The model under review builds one solid part; all positions refer to its coordinate system, in mm. A direction names the side the tool comes from. Coordinates: 2 decimals unless noted, no trailing zeros. Order: outer loops, then holes, each group sorted by start corner. A loop starts at its lowest first (then second) coordinate and runs counter-clockwise, first axis right, second up. Notation, with made-up numbers: (-12, 80.25) - (42, 80.25) arc R17 cw to (42, 94.25) - close; hole circle Ø6 at (9, -6). An arc over 180 degrees is marked (long way). Answer in a Markdown table with one row per item.
```python
from build123d import *

# Parameters (mm, degrees)
ESQUISSE1_W              = 57.9
ESQUISSE1_H              = 86
BOSS_EXTRU_1_DEPTH       = 80
ESQUISSE2_W              = 49.9
ESQUISSE2_H              = 78
ENL_V_MAT_EXTRU_1_DEPTH  = 75
ESQUISSE3_W              = 10
ESQUISSE3_H              = 10
BOSS_EXTRU_2_DEPTH       = 10
ESQUISSE4_R              = 2.75
ENL_V_MAT_EXTRU_2_DEPTH  = 5.85
ESQUISSE47_R             = 2.25
ENL_V_MAT_EXTRU_25_DEPTH = 10
ESQUISSE19_W             = 50
ESQUISSE19_H             = 20
BOSS_EXTRU_9_DEPTH       = 4.75
CONG_1_R                 = 3
ESQUISSE29_W             = 10
ESQUISSE29_H             = 5
ENL_V_MAT_EXTRU_11_DEPTH = 100.346187647
ESQUISSE32_W             = 57.9
ESQUISSE32_H             = 62.5
ENL_V_MAT_EXTRU_16_DEPTH = 4
ESQUISSE46_W             = 3
ESQUISSE46_H             = 5.5
BOSS_EXTRU_10_DEPTH      = 78
ENL_V_START              = -1.5
ENL_V_MAT_EXTRU_20_DEPTH = 11.5
ENL_V_MAT_EXTRU_21_DEPTH = 1.7
CHANFREIN1_SIZE          = 6
ESQUISSE45_R             = 2.75
ENL_V_MAT_EXTRU_24_DEPTH = 100.346187647
ESQUISSE48_W             = 8
ESQUISSE48_H             = 4
BOSS_EXTRU_11_DEPTH      = 15
ESQUISSE49_R             = 2.75
ENL_V_MAT_EXTRU_26_DEPTH = 15
CONG_2_R                 = 2


with BuildPart() as part:
    # Esquisse1 → Boss.-Extru.1 (new body)
    with BuildSketch(Plane.XY):
        Rectangle(ESQUISSE1_W, ESQUISSE1_H)
    extrude(amount=BOSS_EXTRU_1_DEPTH)

    # Esquisse2 → Enlèv. mat.-Extru.1 (cut)
    with BuildSketch(Plane.XY.offset(80)):
        Rectangle(ESQUISSE2_W, ESQUISSE2_H)
    extrude(amount=-ENL_V_MAT_EXTRU_1_DEPTH, mode=Mode.SUBTRACT)

    # Esquisse3 → Boss.-Extru.2 (add)
    with BuildSketch(Plane.XY.offset(80)):
        with Locations((-23.95, 38)):
            Rectangle(ESQUISSE3_W, ESQUISSE3_H)
        with Locations((-23.95, -38)):
            Rectangle(ESQUISSE3_W, ESQUISSE3_H)
        with Locations((23.95, -38)):
            Rectangle(ESQUISSE3_W, ESQUISSE3_H)
        with Locations((23.95, 38)):
            Rectangle(ESQUISSE3_W, ESQUISSE3_H)
    extrude(amount=-BOSS_EXTRU_2_DEPTH)

    # Esquisse4 → Enlèv. mat.-Extru.2 (cut)
    with BuildSketch(Plane.XY.offset(80)):
        with Locations((23.95, -38)):
            Circle(ESQUISSE4_R)
        with Locations((-23.95, -38)):
            Circle(ESQUISSE4_R)
        with Locations((-23.95, 38)):
            Circle(ESQUISSE4_R)
        with Locations((23.95, 38)):
            Circle(ESQUISSE4_R)
    extrude(amount=-ENL_V_MAT_EXTRU_2_DEPTH, mode=Mode.SUBTRACT)

    # Esquisse47 → Enlèv. mat.-Extru.25 (cut)
    with BuildSketch(Plane.XY.offset(80)):
        with Locations((23.95, -38)):
            Circle(ESQUISSE47_R)
        with Locations((-23.95, -38)):
            Circle(ESQUISSE47_R)
        with Locations((-23.95, 38)):
            Circle(ESQUISSE47_R)
        with Locations((23.95, 38)):
            Circle(ESQUISSE47_R)
    extrude(amount=-ENL_V_MAT_EXTRU_25_DEPTH, mode=Mode.SUBTRACT)

    # Esquisse19 → Boss.-Extru.9 (add)
    with BuildSketch(Plane(origin=(0, 0, 0), x_dir=(-1, 0, 0), z_dir=(0, 0, -1))):
        with Locations((0, -7)):
            Rectangle(ESQUISSE19_W, ESQUISSE19_H)
    extrude(amount=BOSS_EXTRU_9_DEPTH)

    # Congé1
    cong_1_edges = [part.edges().sort_by_distance(p)[0] for p in [
        (0, -17, 0),
    ]]
    fillet(cong_1_edges, radius=CONG_1_R)

    # Esquisse29 → Enlèv. mat.-Extru.11 (cut, through all)
    with BuildSketch(Plane(origin=(0, 0, -4.75), x_dir=(-1, 0, 0), z_dir=(0, 0, -1))):
        with Locations((0, -5)):
            Rectangle(ESQUISSE29_W, ESQUISSE29_H)
    extrude(amount=-ENL_V_MAT_EXTRU_11_DEPTH, mode=Mode.SUBTRACT)

    # Esquisse32 → Enlèv. mat.-Extru.16 (cut)
    with BuildSketch(Plane.XZ.offset(43)):
        with Locations((0, 33.25)):
            Rectangle(ESQUISSE32_W, ESQUISSE32_H)
    extrude(amount=-ENL_V_MAT_EXTRU_16_DEPTH, mode=Mode.SUBTRACT)

    # Esquisse46 → Boss.-Extru.10 (add)
    with BuildSketch(Plane.XZ.offset(39)):
        with Locations((-23.45, 15.75)):
            Rectangle(ESQUISSE46_W, ESQUISSE46_H)
    boss_extru_10 = extrude(amount=-BOSS_EXTRU_10_DEPTH)

    # Esquisse38 → Enlèv. mat.-Extru.20 (cut)
    with BuildSketch(Plane(origin=(-24.95, 0, 0), x_dir=(0, 0, -1), z_dir=(1, 0, 0)).offset(ENL_V_START)):
        with BuildLine():
            Line((-16.95, -39), (-16.95, 36))
            ThreePointArc((-16.95, 36), (-15.975, 36.975), (-15, 36))
            Line((-15, 36), (-15, -39))
            ThreePointArc((-15, -39), (-15.975, -39.975), (-16.95, -39))
        make_face()
    enl_v_mat_extru_20 = extrude(amount=ENL_V_MAT_EXTRU_20_DEPTH, mode=Mode.SUBTRACT)

    # Esquisse40 → Enlèv. mat.-Extru.21 (cut)
    with BuildSketch(Plane(origin=(-24.95, 0, 0), x_dir=(0, 0, -1), z_dir=(1, 0, 0))):
        with BuildLine():
            Line((-46.95, 36), (-46.95, -39))
            ThreePointArc((-46.95, -39), (-47.925, -39.975), (-48.9, -39))
            Line((-48.9, -39), (-48.9, 36))
            ThreePointArc((-48.9, 36), (-47.925, 36.975), (-46.95, 36))
        make_face()
    enl_v_mat_extru_21 = extrude(amount=-ENL_V_MAT_EXTRU_21_DEPTH, mode=Mode.SUBTRACT)

    # Chanfrein1
    chanfrein1_edges = [part.edges().sort_by_distance(p)[0] for p in [
        (24.95, -33, 75),
        (-24.95, -33, 75),
        (24.95, 33, 75),
        (-24.95, 33, 75),
    ]]
    chamfer(chanfrein1_edges, length=CHANFREIN1_SIZE - 0.0001)  # a hair under: the kernel refuses the full size

    # Symétrie1: Boss.-Extru.10, Enlèv. mat.-Extru.20, Enlèv. mat.-Extru.21 across plane
    add(boss_extru_10.mirror(Plane(origin=(0, 0, 0), x_dir=(0, 0, 1), z_dir=(1, 0, 0))))
    add(enl_v_mat_extru_20.mirror(Plane(origin=(0, 0, 0), x_dir=(0, 0, 1), z_dir=(1, 0, 0))), mode=Mode.SUBTRACT)
    add(enl_v_mat_extru_21.mirror(Plane(origin=(0, 0, 0), x_dir=(0, 0, 1), z_dir=(1, 0, 0))), mode=Mode.SUBTRACT)

    # Esquisse45 → Enlèv. mat.-Extru.24 (cut, through all)
    with BuildSketch(Plane(origin=(0, 0, -4.75), x_dir=(-1, 0, 0), z_dir=(0, 0, -1))):
        with Locations((17, -6)):
            Circle(ESQUISSE45_R)
        with Locations((-17, -6)):
            Circle(ESQUISSE45_R)
    extrude(amount=-ENL_V_MAT_EXTRU_24_DEPTH, mode=Mode.SUBTRACT)

    # Esquisse48 → Boss.-Extru.11 (add)
    with BuildSketch(Plane.XZ.offset(39)):
        with Locations((0, 7)):
            Rectangle(ESQUISSE48_W, ESQUISSE48_H)
    extrude(amount=-BOSS_EXTRU_11_DEPTH)

    # Esquisse49 → Enlèv. mat.-Extru.26 (cut)
    with BuildSketch(Plane.XZ.offset(39)):
        with Locations(Location((0, 5.5, 0), (0, 0, 270))):
            Circle(ESQUISSE49_R)
    extrude(amount=-ENL_V_MAT_EXTRU_26_DEPTH, mode=Mode.SUBTRACT)

    # Congé2
    cong_2_edges = [part.edges().sort_by_distance(p)[0] for p in [
        (4, -31.5, 5),
        (-4, -31.5, 5),
    ]]
    fillet(cong_2_edges, radius=CONG_2_R)
    cong_2_2_edges = [part.edges().sort_by_distance(p)[0] for p in [
        (4, -31.5, 9),
        (-4, -31.5, 9),
    ]]
    fillet(cong_2_2_edges, radius=CONG_2_R - 0.0001)  # a hair under: the kernel refuses the full size


solid = part.part
```
Item 1: Mouldability with a two-part tool opening along Y and no side actions: class faces 6 (the face through (23, -1, 13)), 7 (the face through (2, -39, 8)), 8 (the face through (18.95, 36, 75)) as +Y half, -Y half, draft (parallel to the pull), parting line (faces both ways), or undercut.
Check values:
| item | result |
|---|---|
| face 6 | draft |
| face 7 | -Y half |
| face 8 | undercut |
Item 2: We need section D-D, the plane z = 68. Write out the cut boundary in (x, y).
Check values:
| item | result |
|---|---|
| outline | (-28.95, -43) - (28.95, -43) - (28.95, 43) - (-28.95, 43) - close; hole (-24.95, -39) - (24.95, -39) - (24.95, 39) - (-24.95, 39) - close |
Item 3: We need section C-C, the plane z = 54.5. Write out the cut boundary in (x, y).
Check values:
| item | result |
|---|---|
| outline | (-28.95, -39) - (-24.95, -39) - (-24.95, 39) - (24.95, 39) - (24.95, -39) - (28.95, -39) - (28.95, 43) - (-28.95, 43) - close |
Item 4: We need section B-B, the plane x = 0. Write out the cut boundary in (y, z), then the cut area to 3 significant figures.
Check values:
| item | result |
|---|---|
| outline | (-43, 0) - (-20, 0) arc R3 cw to (-17, -3) - (-17, -4.75) - (-7.5, -4.75) - (-7.5, 5) - (-24, 5) - (-24, 2.75) - (-39, 2.75) - (-39, 2) - (-43, 2) - close; (-43, 64.5) - (-39, 64.5) - (-39, 80) - (-43, 80) - close; (-39, 8.25) - (-24, 8.25) - (-24, 9) - (-39, 9) - close; (-2.5, -4.75) - (3, -4.75) - (3, 0) - (43, 0) - (43, 80) - (39, 80) - (39, 5) - (-2.5, 5) - close |
| area | 806 mm^2 |
Item 5: We need section A-A, the plane x = 17. Write out the cut boundary in (y, z), then the cut area to 3 significant figures.
Check values:
| item | result |
|---|---|
| outline | (-43, 0) - (-20, 0) arc R3 cw to (-17, -3) - (-17, -4.75) - (-8.75, -4.75) - (-8.75, 5) - (-39, 5) - (-39, 2) - (-43, 2) - close; (-43, 64.5) - (-39, 64.5) - (-39, 80) - (-43, 80) - close; (-3.25, -4.75) - (3, -4.75) - (3, 0) - (43, 0) - (43, 80) - (39, 80) - (39, 5) - (-3.25, 5) - close |
| area | 823 mm^2 |
Item 6: Tool access review of faces 1 (the face through (-18.95, 36, 75)), 2 (the face through (0, -41, 2)), 3 (the face through (-23, -1, 13)), 4 (the face through (-22, -33, 70)), 5 (the face through (-25, -6, -2)): name each direction out of +Z, -Z, +X, -X, +Y, -Y from which nothing blocks a thin tool from reaching the whole face with its end or side.
Check values:
| item | result |
|---|---|
| face 1 | +Z |
| face 2 | +X, -X, -Y |
| face 3 | -Y |
| face 4 | none |
| face 5 | -Z, -X, +Y, -Y |
Item 7: To check wall thickness, follow line 1 (X direction, y = 38, z = 72); line 2 (Z direction, x = -23, y = -20.5); line 3 (Z direction, x = 24.5, y = -35). State the ranges of each line that lie inside material, in increasing order. Write a range as from..to.
Check values:
| item | result |
|---|---|
| line 1 | -28.95..-26.2, -21.7..-18.95, 18.95..21.7, 26.2..28.95 |
| line 2 | 0..5, 13..15, 16.95..18.5 |
| line 3 | 0..5, 13..15, 16.95..18.5, 70..80 |
Item 8: Clearance check with flat-ended pins moving along their axes: pin 1 Ø2.5 at (x, y) = (-23.95, -38) entering from +Z; pin 2 Ø12 at (x, y) = (-11, 4.5) entering from +Z; pin 3 Ø10.5 at (x, z) = (1, -0.5) entering from +Y; pin 4 Ø0.9 at (x, y) = (23.5, 6) entering from +Z. State where each tip first meets the part, or that it passes through.
Check values:
| item | result |
|---|---|
| pin 1 | z = 70 |
| pin 2 | z = 5 |
| pin 3 | y = 43 |
| pin 4 | z = 18.5 |
